For this review, take the finished solid that the model builds, in its own axes (mm). Coordinates: 2 decimals unless noted, no trailing zeros. Write each loop counter-clockwise with the first axis right and the second up, starting at its lowest first coordinate (ties: lowest second). Pieces come first, ordered by that corner, then holes. Notation, with made-up numbers: (-25.5, -3.5) - (13.5, -3.5) arc R19 ccw to (13.5, 12.5) - close; hole circle Ø3 at (-40, 58). An arc over 180 degrees is marked (long way). Write each question's results on one line, items separated by ' | '.
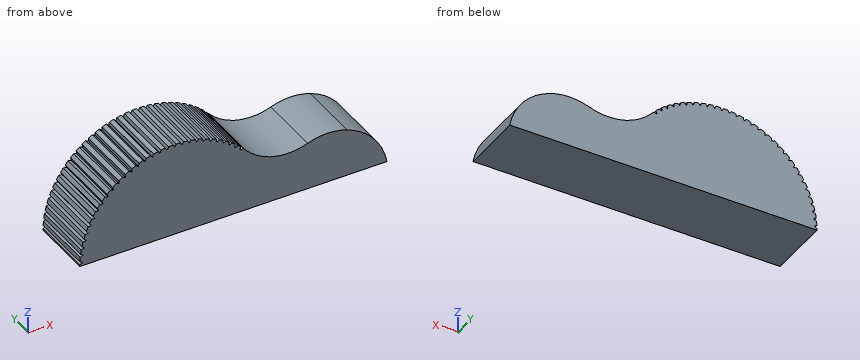
from build123d import *

# Parameters (mm, degrees)
F1_DEPTH         = 5.5
F3_DEPTH         = 5.501
F3_COPIES_COUNT  = 20
F3_COPIES_ANGLE  = 88.0004
F3_COPIES1_COUNT = 11
F3_COPIES1_ANGLE = 45


# Not quite as in the source:
# - a pattern or mirror of a feature is missing from the dataset's text; its kind, count and spacing are read off the source's solid


with BuildPart() as f1:
    # F0 (on Front) → F1 (new body)
    with BuildSketch(Plane.XZ):
        with BuildLine():
            Line((-27, 0), (0, 0))
            ThreePointArc((0, 0), (-1.1926360457, 2.5804184186), (-3.5143684573, 4.2206923475))
            ThreePointArc((-3.5143684573, 4.2206923475), (-5.2460959941, 4.5301572247), (-6.977823531, 4.2206923475))
            ThreePointArc((-6.977823531, 4.2206923475), (-9.9132769797, 4.0582856894), (-12.4325656492, 5.5736890919))
            ThreePointArc((-12.4325656492, 5.5736890919), (-21.6338668847, 7.7986561929), (-27, 0))
        make_face()
    extrude(amount=F1_DEPTH)

    # F2 (on face) → F3 (cut, through all)
    with BuildSketch(Plane.XZ.offset(5.5)):
        with BuildLine():
            ThreePointArc((-18.5063756326, 8.3487647015), (-18.65, 8.35), (-18.7936243674, 8.3487647015))
            Line((-18.7936243674, 8.3487647015), (-18.65, 8.1))
            Line((-18.65, 8.1), (-18.5063756326, 8.3487647015))
        make_face()
    f3 = extrude(amount=-F3_DEPTH, mode=Mode.SUBTRACT)

    # F3_copies: F3 ×20 about axis
    f3_copies_axis = Axis((-18.65, 0, 0), (0, -1, 0))
    for i in range(1, F3_COPIES_COUNT):
        add(f3.rotate(f3_copies_axis, i * F3_COPIES_ANGLE / (F3_COPIES_COUNT - 1)), mode=Mode.SUBTRACT)

    # F3_copies1: F3 ×11 about axis
    f3_copies1_axis = Axis((-18.65, 0, 0), (0, 1, 0))
    for i in range(1, F3_COPIES1_COUNT):
        add(f3.rotate(f3_copies1_axis, i * F3_COPIES1_ANGLE / (F3_COPIES1_COUNT - 1)), mode=Mode.SUBTRACT)


solid = f1.part
Q1. For pin 1 (1 mm diameter, centred on y = -4.5, z = 5.5, fed in from -X); pin 2 (3 mm diameter, centred on x = -11.5, z = 6, fed in from +Y); pin 3 (3 mm diameter, centred on y = -4, z = 3.5, fed in from +X); pin 4 (2 mm diameter, centred on y = -5, z = 2, fed in from -X), all flat-tipped, find the tip position at first contact; note any pin that passes through.
Results found:
pin 1: x = -25.34 | pin 2: y = 0 | pin 3: x = -0.77 | pin 4: x = -26.93
Q2. Wall thickness on line 1 along Z through (x, y) = (-5.25, -1); line 2 along Z through (x, y) = (-15.75, -1.65); line 3 along X through (y, z) = (-4.55, 1): over which ranges is each line inside the solid? List them lowest first. Write a range as from..to.
Results found:
line 1: 0..4.53 | line 2: 0..7.83 | line 3: -26.78..-0.27
Q3. Take a section at A-A on x = -11.75. State the section outline as (y, z) points, plus the area to 3 significant figures.
Results found:
outline: (-5.5, 0) - (0, 0) - (0, 4.94) - (-5.5, 4.94) - close | area: 27.2 mm2
